The figure shows three views and two pictorial views of one solid part (mm, origin at its lowest corner). Answer the questions. Coordinates: 2 decimals unless noted, no trailing zeros. Loops run counter-clockwise (first coordinate to the right, second up) from the corner with the lowest first, then second, coordinate; pieces in that order, holes last. Notation, with made-up numbers: M 89.25,28 L 139.25,28 A27 ccw 139.25,57 Z; hole C -4,-31 d8. An arc over 180 degrees is marked long. Return JSON: item names as keys, results as strings. Group by question number.
1. Section C-C (x = 21) is taken. Write down the section's boundary in (y, z), then the cut area to 3 significant figures.
2. Section D-D (y = 37) is taken. Write down the section's boundary in (x, z).
3. Given P1, Ø1.1, axis at x = 1.5, z = 1.5, coming from the +Y side; P2, Ø1.5, axis at y = 5.5, z = 1, coming from the +X side; P3, Ø1, axis at x = 39, y = 34.5, coming from the +Z side, each flat-ended and moving along its own axis, determine where each tip first touches the part or whether it passes through.
4. Section B-B (z = 1.75) is taken. Write down the section's boundary in (x, y).
5. Straight lines are drawn through the part: L1, parallel to Y at x = 21, z = 1.3; L2, parallel to X at y = 40, z = 1.8; L3, parallel to X at y = 28, z = 0.3. For each, find the intervals that lie inside material, in ascending order. Write a range as from..to.
6. Section A-A (y = 29) is taken. Write down the section's boundary in (x, z).
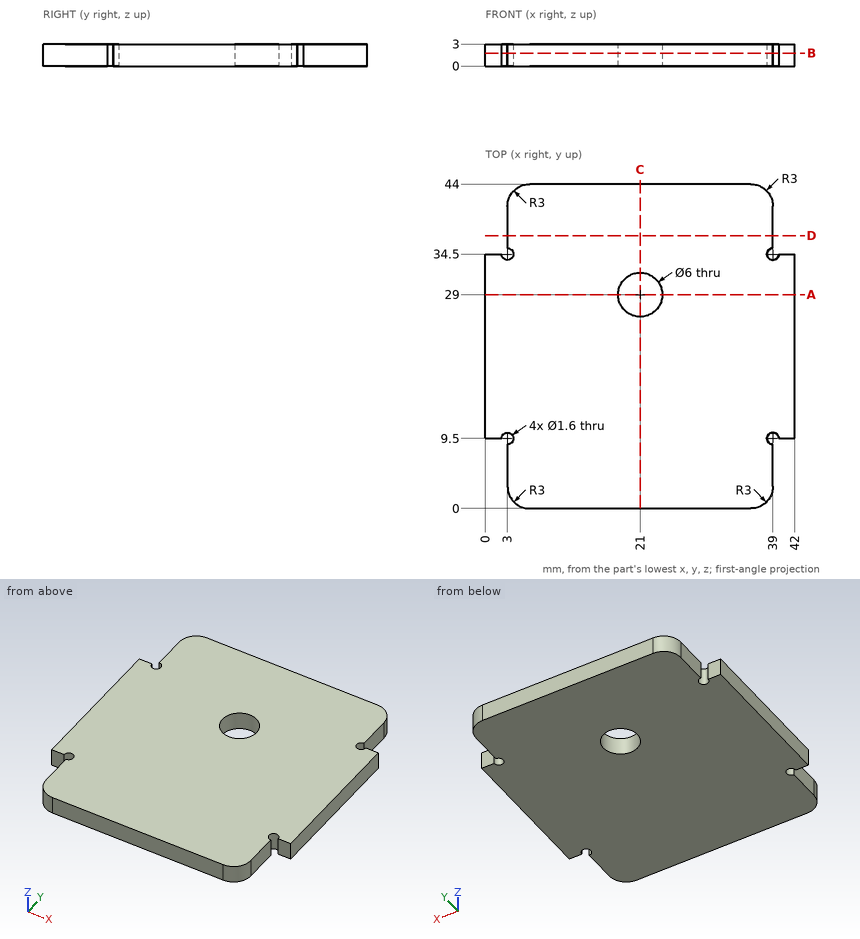
Worked out:
{
 "1": {"outline": "M 0,0 L 26,0 L 26,3 L 0,3 Z; M 32,0 L 44,0 L 44,3 L 32,3 Z", "area": "114 mm^2"},
 "2": {"outline": "M 3,0 L 39,0 L 39,3 L 3,3 Z"},
 "3": {"P1": "y = 34.5", "P2": "x = 39", "P3": "through"},
 "4": {"outline": "M 0,9.5 L 2.2,9.5 A0.8 cw long 3,8.7 L 3,3 A3 ccw 6,0 L 36,0 A3 ccw 39,3 L 39,8.7 A0.8 cw long 39.8,9.5 L 42,9.5 L 42,34.5 L 39.8,34.5 A0.8 cw long 39,35.3 L 39,41 A3 ccw 36,44 L 6,44 A3 ccw 3,41 L 3,35.3 A0.8 cw long 2.2,34.5 L 0,34.5 Z; hole C 21,29 d6"},
 "5": {"L1": "0..26, 32..44", "L2": "3..39", "L3": "0..18.17, 23.83..42"},
 "6": {"outline": "M 0,0 L 18,0 L 18,3 L 0,3 Z; M 24,0 L 42,0 L 42,3 L 24,3 Z"}
}
